Geometry: final body of the model. Coordinates: model frame, mm. A direction names the side the tool comes from. Round coordinates to 2 decimals unless told otherwise and drop trailing zeros. Order: outer loops, then holes, each group sorted by start corner. A loop starts at its lowest first (then second) coordinate and runs counter-clockwise, first axis right, second up. Notation, with made-up numbers: M -1,84.25 L 26,84.25 A15 cw 26,113.25 Z; hole C 16,52 d3. An arc over 180 degrees is marked long. Return JSON: item names as keys, results as strings. Group by question number.
Q1. Cut plane D-D on z = 2. Output: boundary loops of the cut face in (x, y).
Q2. Contact query for a flat-ended pin moving along its axis: pin 1 (3 mm diameter, centred on y = 3, z = 3, fed in from +X). Output: stop coordinate, or through.
Q3. Cut plane C-C on x = 0. Output: boundary loops of the cut face in (y, z), and give its area (3 significant figures).
Q4. Cut plane A-A on z = 8. Output: boundary loops of the cut face in (x, y).
Q5. Cut plane B-B on y = 0. Output: boundary loops of the cut face in (x, z).
Q6. Mould query, pull axis X, two halves, no side actions, for faces 3 (the face through (6, 0, 5)), 4 (the face through (-0.867, -3.905, 8.028)), 5 (the face through (-6, 0, 5)). Classes: released by +X, released by -X, zero draft, split by the parting line, or undercut.
Q7. Ray query, probe 1 along Y at (x, z) = (0, 7.25); probe 2 along Y at (x, z) = (3, 5); probe 3 along Y at (x, z) = (0, 3.8). Return the intervals inside material, ascending.
Q8. Access query for faces 1 (the face through (2, 0, 6)), 2 (the face through (-1.4, 4.1, 10)). Directions: +Z, -Z, +X, -X, +Y, -Y. A direction counts if a zero-diameter tool reaches every point of the face in a straight line with its end or side. Return the directions, or none.
```python
from build123d import *

# Parameters (mm, degrees)
EXTRUDE_1_DEPTH     = 10
SKETCH_2_R          = 4
CUT_EXTRUDE_1_DEPTH = 4
M4X0_71_D           = 3.3
FILLET_1_R          = 1.5


with BuildPart() as part:
    # Эскиз1 → Бобышка-Вытянуть1 (new body)
    with BuildSketch(Plane.XY):
        with BuildLine():
            Line((0, 10), (-4.8, 3.6))
            ThreePointArc((-4.8, 3.6), (-6, 0), (-4.8, -3.6))
            Line((-4.8, -3.6), (0, -10))
            Line((0, -10), (4.8, -3.6))
            ThreePointArc((4.8, -3.6), (6, 0), (4.8, 3.6))
            Line((4.8, 3.6), (0, 10))
        make_face()
    extrude(amount=EXTRUDE_1_DEPTH)

    # Эскиз2 → Вырез-Вытянуть1 (cut)
    with BuildSketch(Plane.XY.offset(10)):
        Circle(SKETCH_2_R)
    extrude(amount=-CUT_EXTRUDE_1_DEPTH, mode=Mode.SUBTRACT)

    # Отверстие обработанное метчиком M4x0.71 (through all)
    with Locations(Plane.XY.offset(6)):
        with Locations((0, 0)):
            Hole(M4X0_71_D / 2)

    # Скругление1
    fillet_1_edges = [part.edges().sort_by_distance(p)[0] for p in [
        (0, -10, 5),
        (0, 10, 5),
    ]]
    fillet(fillet_1_edges, radius=FILLET_1_R)


solid = part.part
```
Result sheet:
{
 "1": {"outline": "M -4.8,-3.6 L -1.2,-8.4 A1.5 ccw 1.2,-8.4 L 4.8,-3.6 A6 ccw 4.8,3.6 L 1.2,8.4 A1.5 ccw -1.2,8.4 L -4.8,3.6 A6 ccw Z; hole C 0,0 d3.3"},
 "2": {"pin 1": "stops at x = 5.81"},
 "3": {"outline": "M -9,0 L -1.65,0 L -1.65,6 L -4,6 L -4,10 L -9,10 Z; M 1.65,0 L 9,0 L 9,10 L 4,10 L 4,6 L 1.65,6 Z", "area": "128 mm²"},
 "4": {"outline": "M -4.8,-3.6 L -1.2,-8.4 A1.5 ccw 1.2,-8.4 L 4.8,-3.6 A6 ccw 4.8,3.6 L 1.2,8.4 A1.5 ccw -1.2,8.4 L -4.8,3.6 A6 ccw Z; hole C 0,0 d8"},
 "5": {"outline": "M -6,0 L -1.65,0 L -1.65,6 L -4,6 L -4,10 L -6,10 Z; M 1.65,0 L 6,0 L 6,10 L 4,10 L 4,6 L 1.65,6 Z"},
 "6": {"face 3": "released by +X", "face 4": "undercut", "face 5": "released by -X"},
 "7": {"probe 1": "y = -9 to -4, 4 to 9", "probe 2": "y = -6 to 6", "probe 3": "y = -9 to -1.65, 1.65 to 9"},
 "8": {"face 1": "+Z", "face 2": "+Z, +X, -X, +Y, -Y"}
}
